```python
from build123d import *

# Parameters (mm, degrees)
SKETCH_1_W                   = 12
SKETCH_1_H                   = 8
EXTRUDE_1_DEPTH              = 595
HOLE_WIZARD_M3_1_D           = 3.4
HOLE_WIZARD_M3_1_CBORE_D     = 6.5
HOLE_WIZARD_M3_1_CBORE_DEPTH = 3.4
PATTERN_LINEAR_1_COUNT       = 24
PATTERN_LINEAR_1_PITCH       = 25


with BuildPart() as part:
    # 草图1 → 凸台-拉伸1 (new body)
    with BuildSketch(Plane.XY):
        with Locations((6, 4)):
            Rectangle(SKETCH_1_W, SKETCH_1_H)
    extrude(amount=EXTRUDE_1_DEPTH)

    # M3 六角凹头螺钉的柱形沉头孔1 (through all)
    with Locations(Plane(origin=(0, 8, 0), x_dir=(1, 0, 0), z_dir=(0, 1, 0))):
        with Locations((6, -585)):
            hole_wizard_m3_1 = CounterBoreHole(HOLE_WIZARD_M3_1_D / 2, HOLE_WIZARD_M3_1_CBORE_D / 2, HOLE_WIZARD_M3_1_CBORE_DEPTH)

    # 阵列(线性)1: M3 六角凹头螺钉的柱形沉头孔1 ×24
    with Locations(*[(0, 0, -i * PATTERN_LINEAR_1_PITCH) for i in range(1, PATTERN_LINEAR_1_COUNT)]):
        add(hole_wizard_m3_1, mode=Mode.SUBTRACT)


solid = part.part
```
Part model, mm, in its own coordinate system. Give positions to 0.01 mm unless a question says otherwise; leave off trailing zeros. Return JSON: item names as keys, results as strings.
1) Drill centre lines: line 1 (X direction, y = 3.2, z = 10); line 2 (X direction, y = 5.5, z = 335). Where is each one in solid material? Low to high.
Calculated:
{"line 1": "x = 0 to 4.3, 7.7 to 12", "line 2": "x = 0 to 2.75, 9.25 to 12"}
2) Flat gauge pins, fed straight in: pin 1 Ø2 at (x, z) = (11, 412) entering from -Y; pin 2 Ø5.5 at (x, z) = (6, 510) entering from +Y; pin 3 Ø2.5 at (x, z) = (6, 385) entering from +Y. Where does each tip first touch, or does it go through?
Calculated:
{"pin 1": "stops at y = 0", "pin 2": "stops at y = 4.6", "pin 3": "passes through"}
3) Saw through at A-A, the plane y = 3. Count the separate pieces of the cut face and the enclosed holes in it, then the cut area to 3 significant figures.
Calculated:
{"separate pieces": "1", "enclosed holes": "24", "area": "6,920 mm2"}
